from build123d import *

# Parameters (mm, degrees)
F0_R      = 74.6125
F1_DEPTH  = 19.05
F2_R      = 50.8
F3_DEPTH  = 88.9
F4_R      = 74.6125
F5_DEPTH  = 19.05
F6_R      = 7.14375
F7_DEPTH  = 127.001
F8_R      = 38.1
F9_DEPTH  = 3.175
F10_R     = 38.1
F11_DEPTH = 120.65
F12_SIZE  = 1.905


with BuildPart() as f1:
    # F0 (on Top) → F1 (new body)
    with BuildSketch(Plane.XY):
        Circle(F0_R)
    extrude(amount=F1_DEPTH)

    # F2 (on face) → F3 (join)
    with BuildSketch(Plane.XY.offset(19.05)):
        Circle(F2_R)
    extrude(amount=F3_DEPTH)

    # F4 (on face) → F5 (join)
    with BuildSketch(Plane.XY.offset(107.95)):
        Circle(F4_R)
    extrude(amount=F5_DEPTH)

    # F6 (on face) → F7 (cut, through all)
    with BuildSketch(Plane.XY.offset(127)):
        with Locations((24.5654228837, 58.5558707436)):
            Circle(F6_R)
        with Locations((-38.4281601629, 50.5522156438)):
            Circle(F6_R)
        with Locations((-62.9935830465, -8.0036550999)):
            Circle(F6_R)
        with Locations((-24.5654228837, -58.5558707436)):
            Circle(F6_R)
        with Locations((38.4281601629, -50.5522156438)):
            Circle(F6_R)
        with Locations((62.9935830465, 8.0036550999)):
            Circle(F6_R)
    extrude(amount=-F7_DEPTH, mode=Mode.SUBTRACT)

    # F8 (on face) → F9 (join)
    with BuildSketch(Plane.XY.offset(127)):
        Circle(F8_R)
    extrude(amount=F9_DEPTH)

    # F10 (on face) → F11 (cut)
    with BuildSketch(Plane(origin=(0, 0, 0), x_dir=(1, 0, 0), z_dir=(0, 0, -1))):
        Circle(F10_R)
    extrude(amount=-F11_DEPTH, mode=Mode.SUBTRACT)

    # F12
    f12_edges = [f1.edges().sort_by_distance(p)[0] for p in [
        (-74.6125, 0, 0),
        (-38.1, 0, 0),
        (-74.6125, 0, 19.05),
        (-74.6125, 0, 107.95),
        (-74.6125, 0, 127),
        (-38.1, 0, 130.175),
    ]]
    chamfer(f12_edges, length=F12_SIZE)


solid = f1.part
Verification items for the finished model (mm, model axes). A direction names the side the tool comes from. Give positions to 0.01 mm unless a question says otherwise; leave off trailing zeros. Loops run counter-clockwise (first coordinate to the right, second up) from the corner with the lowest first, then second, coordinate; pieces in that order, holes last. Notation, with made-up numbers: (43, -5.5) - (69, -5.5) arc R26 cw to (69, 29.5) - close; hole circle Ø10 at (-20, 39). An arc over 180 degrees is marked (long way). Write each question's results on one line, items separated by ' | '.
1) Sectioned sample at C-C on y = 5.5. Count the separate pieces of the cut face and the enclosed holes in it, plus the area to 3 significant figures.
Solution:
separate pieces: 3 | enclosed holes: 0 | area: 5,260 mm2
2) Mould release check, pull along Y, two halves, no side actions. Record for faces 1 (the cylindrical face through (-11.012, -49.592, 62.878)), 2 (the cylindrical face through (-56.18, -5.86, 117.61)), 3 (the flat face through (31, -31, 127)): pulls with the +Y half, pulls with the -Y half, needs draft (parallel to the pull), parting line crosses it, or undercut.
Solution:
face 1: parting line crosses it | face 2: undercut | face 3: needs draft
3) Depth check by flat-ended pin: P1, Ø6, axis at x = 8.5, y = 28, coming from the -Z side; P2, Ø18.5, axis at x = 24.57, y = 58.56, coming from the +Z side; P3, Ø8, axis at x = -51, z = 70, coming from the -Y side. Enter the tip coordinate at first touch or a pass-through.
Solution:
P1: z = 120.65 | P2: z = 127 | P3: y = -19.28
4) Sectioned sample at B-B on z = 31.5. Record the boundary of the cut face in (x, y).
Solution:
outline: circle Ø101.6 at (0, 0); hole circle Ø76.2 at (0, 0)
5) Material ranges on L1, parallel to Z at x = -62.5, y = -26; L2, parallel to Z at x = 19, y = 7.5 (3 decimals); L3, parallel to X at y = 33, z = 25.5, recorded low to high. Write a range as from..to.
Solution:
L1: 0..19.05, 107.95..127 | L2: 120.65..130.175 | L3: -38.62..-19.04, 19.04..38.62
6) Tool access check on faces 4 (the cylindrical face through (27.862, 52.218, 9.658)), 5 (the cylindrical face through (-30.235, 23.183, 60.446)), 6 (the conical face through (-15.787, -71.095, 18.931)). Record the directions out of +Z, -Z, +X, -X, +Y, -Y that give a thin tool (end or side, any length) a straight path to the whole face; none if there is none.
Solution:
face 4: +Z, -Z | face 5: -Z | face 6: none
